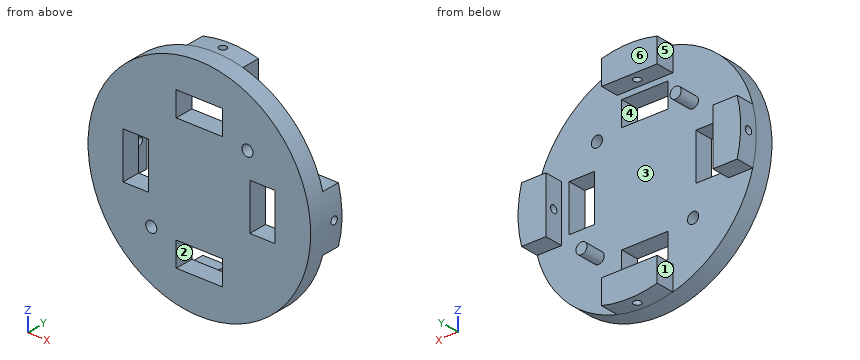
```python
from build123d import *

# Parameters (mm, degrees)
SKETCH1_R           = 76.2
BOSS_EXTRUDE1_DEPTH = 12.7
SKETCH9_W           = 17.40446846
SKETCH9_H           = 31.75
SKETCH9_W_2         = 17.404468459
SKETCH9_W_3         = 31.75
SKETCH9_H_2         = 16.793136505
CUT_EXTRUDE1_DEPTH  = 12.7
SKETCH12_R          = 3.81
CUT_EXTRUDE7_DEPTH  = 13.7
SKETCH14_R          = 3.81
BOSS_EXTRUDE5_DEPTH = 13.97
BOSS_EXTRUDE6_DEPTH = 12.7
SKETCH15_R          = 2.5654
CUT_EXTRUDE8_DEPTH  = 20.05
CIRPATTERN1_COUNT   = 4


with BuildPart() as part:
    # Sketch1 → Boss-Extrude1 (new body)
    with BuildSketch(Plane(origin=(0, 0, 0), x_dir=(1, 0, 0), z_dir=(0, 1, 0))):
        Circle(SKETCH1_R)
    extrude(amount=BOSS_EXTRUDE1_DEPTH)

    # Sketch9 → Cut-Extrude1 (cut)
    with BuildSketch(Plane(origin=(0, 12.7, 0), x_dir=(1, 0, 0), z_dir=(0, 1, 0))):
        with Locations((43.222256972, -1.420690531)):
            Rectangle(SKETCH9_W, SKETCH9_H)
        with Locations((-43.511171149, -1.420690531)):
            Rectangle(SKETCH9_W_2, SKETCH9_H)
        with Locations((0.046278064, 44.665088999)):
            Rectangle(SKETCH9_W_3, SKETCH9_H_2)
        with Locations((0.046278064, -45.105910611)):
            Rectangle(SKETCH9_W_3, SKETCH9_H_2)
    extrude(amount=-CUT_EXTRUDE1_DEPTH, mode=Mode.SUBTRACT)

    # Sketch12 → Cut-Extrude7 (cut, through all)
    with BuildSketch(Plane(origin=(0, 12.7, 0), x_dir=(1, 0, 0), z_dir=(0, 1, 0))):
        with Locations((-32.923159658, 34.412296975)):
            Circle(SKETCH12_R)
        with Locations((32.923159658, -34.412296975)):
            Circle(SKETCH12_R)
    extrude(amount=-CUT_EXTRUDE7_DEPTH, mode=Mode.SUBTRACT)

    # Sketch14 → Boss-Extrude5 (add)
    with BuildSketch(Plane(origin=(0, 12.7, 0), x_dir=(1, 0, 0), z_dir=(0, 1, 0))):
        with Locations((31.714292366, 35.529484723)):
            Circle(SKETCH14_R)
        with Locations((-32.761256964, -34.580899947)):
            Circle(SKETCH14_R)
    extrude(amount=BOSS_EXTRUDE5_DEPTH)

    # Sketch2 → Boss-Extrude6 (add)
    with BuildSketch(Plane(origin=(0, 12.7, 0), x_dir=(1, 0, 0), z_dir=(0, 1, 0))):
        with BuildLine():
            Line((-19.05, -57.15), (-19.05, -73.780332745))
            ThreePointArc((-19.05, -73.780332745), (0, -76.2), (19.05, -73.780332745))
            Line((19.05, -73.780332745), (19.05, -57.15))
            Line((19.05, -57.15), (-19.05, -57.15))
        make_face()
    boss_extrude6 = extrude(amount=BOSS_EXTRUDE6_DEPTH)

    # Sketch15 → Cut-Extrude8 (cut, through all)
    with BuildSketch(Plane(origin=(0, 0, 57.15), x_dir=(-1, 0, 0), z_dir=(0, 0, -1))):
        with Locations((0, 19.05)):
            Circle(SKETCH15_R)
    cut_extrude8 = extrude(amount=-CUT_EXTRUDE8_DEPTH, mode=Mode.SUBTRACT)

    # CirPattern1: Boss-Extrude6, Cut-Extrude8 ×4 about axis
    cirpattern1_axis = Axis((0, 0, 0), (0, 1, 0))
    for i in range(1, CIRPATTERN1_COUNT):
        add(boss_extrude6.rotate(cirpattern1_axis, i * 360 / CIRPATTERN1_COUNT))
        add(cut_extrude8.rotate(cirpattern1_axis, i * 360 / CIRPATTERN1_COUNT), mode=Mode.SUBTRACT)


solid = part.part
```
Here's how the part is built. I have some questions about the finished solid (model axes, mm). Face numbers are marked on the shaded views. A direction names the side the tool comes from. Coordinates: 2 decimals unless noted, no trailing zeros. Order: outer loops, then holes, each group sorted by start corner. A loop starts at its lowest first (then second) coordinate and runs counter-clockwise, first axis right, second up.
1) We'd pull the mould along X, two halves only. Please class the marked faces 4, 5 and 6: +X half, -X half, draft (parallel to the pull), parting line (faces both ways), or undercut.
2) I need wall thicknesses on line 1 (Y direction, x = 0, z = -69.25); line 2 (X direction, y = 19.05, z = -63.75); line 3 (Z direction, x = 7.5, y = 2.25). Which ranges of each line are inside material? Lowest first, please.
3) Imagine slicing it at B-B on x = 0. List the corners of the cut face in (y, z) for me.
4) Will these pins go through, and if not, where does the flat tip stop? pin 1 (9.5 mm diameter, centred on x = -71, z = -7.5, fed in from +Y); pin 2 (6.5 mm diameter, centred on y = 5.5, z = 6, fed in from -X); pin 3 (4 mm diameter, centred on x = 19.5, y = 13, fed in from -Z).
5) Imagine slicing it at A-A on z = 0. List the corners of the cut face in (x, y) for me, and give its area (3 significant figures).
6) Imagine slicing it at C-C on y = 5.5. List the corners of the cut face in (x, z) for me, and give its area (3 significant figures).
7) Which directions (+Z, -Z, +X, -X, +Y, -Y) give clear straight access to the entire face, cutting with the end or side of a thin tool? Please do the marked faces 1, 2 and 3.
8) Imagine slicing it at D-D on x = 39. List the corners of the cut face in (y, z) for me, and give its area (3 significant figures).
Response values:
1. face 4: undercut
1. face 5: -X half
1. face 6: draft
2. line 1: y = 0 to 16.48, 21.62 to 25.4
2. line 2: x = -19.05 to -2.57, 2.57 to 19.05
2. line 3: z = -75.83 to -53.06, -36.27 to 36.71, 53.5 to 75.83
3. outline: (0, -76.2) - (16.48, -76.2) - (16.48, -57.15) - (12.7, -57.15) - (12.7, -53.06) - (0, -53.06) - close; (0, -36.27) - (12.7, -36.27) - (12.7, 36.71) - (0, 36.71) - close; (0, 53.5) - (12.7, 53.5) - (12.7, 57.15) - (16.48, 57.15) - (16.48, 76.2) - (0, 76.2) - close; (21.62, -76.2) - (25.4, -76.2) - (25.4, -57.15) - (21.62, -57.15) - close; (21.62, 57.15) - (25.4, 57.15) - (25.4, 76.2) - (21.62, 76.2) - close
4. pin 1: stops at y = 25.4
4. pin 2: stops at x = -76.15
4. pin 3: stops at z = -74.16
5. outline: (-76.2, 0) - (-52.21, 0) - (-52.21, 12.7) - (-57.15, 12.7) - (-57.15, 16.48) - (-76.2, 16.48) - close; (-76.2, 21.62) - (-57.15, 21.62) - (-57.15, 25.4) - (-76.2, 25.4) - close; (-34.81, 0) - (34.52, 0) - (34.52, 12.7) - (-34.81, 12.7) - close; (51.92, 0) - (76.2, 0) - (76.2, 16.48) - (57.15, 16.48) - (57.15, 12.7) - (51.92, 12.7) - close; (57.15, 21.62) - (76.2, 21.62) - (76.2, 25.4) - (57.15, 25.4) - close
5. area: 1,780 mm2
6. outline: circle Ø152.4 at (0, 0); hole (-52.21, -14.45) - (-34.81, -14.45) - (-34.81, 17.3) - (-52.21, 17.3) - close; hole circle Ø7.62 at (-32.92, -34.41); hole (-15.83, -53.06) - (15.92, -53.06) - (15.92, -36.27) - (-15.83, -36.27) - close; hole (-15.83, 36.71) - (15.92, 36.71) - (15.92, 53.5) - (-15.83, 53.5) - close; hole circle Ø7.62 at (32.92, 34.41); hole (34.52, -14.45) - (51.92, -14.45) - (51.92, 17.3) - (34.52, 17.3) - close
6. area: 16,000 mm2
7. face 1: +Z, -Z, -X, +Y
7. face 2: +Y, -Y
7. face 3: +Y
8. outline: (0, -65.46) - (12.7, -65.46) - (12.7, -14.45) - (0, -14.45) - close; (0, 17.3) - (12.7, 17.3) - (12.7, 65.46) - (0, 65.46) - close
8. area: 1,260 mm2
